Can you work these out from the model? Positions are in its coordinate system, mm. Face numbers are marked on the shaded views. A direction names the side the tool comes from. Round coordinates to 2 decimals unless told otherwise and drop trailing zeros. Order: outer loops, then holes, each group sorted by start corner. A loop starts at its lowest first (then second) coordinate and runs counter-clockwise, first axis right, second up.
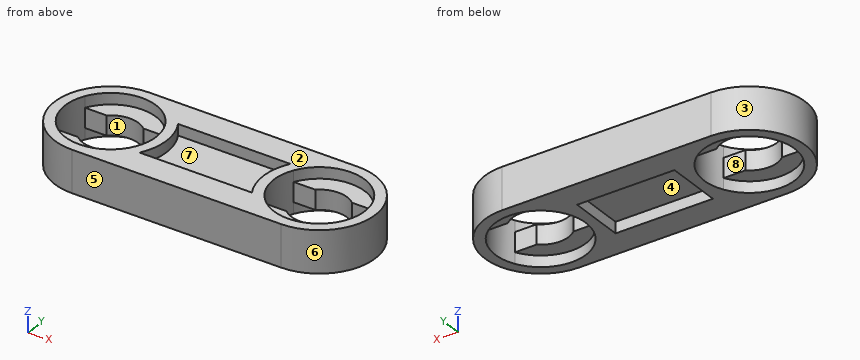
from build123d import *

# Parameters (mm, degrees)
EXTRUDE_1_DEPTH     = 3
CUT_EXTRUDE_1_REACH = 21.647
SKETCH_3_R          = 3.25
CUT_EXTRUDE_2_DEPTH = 0.8
CUT_EXTRUDE_START   = -2.2
SKETCH_3_2_R        = 3.25
CUT_EXTRUDE_3_DEPTH = 0.8
CUT_EXTRUDE_4_DEPTH = 0.8
SKETCH_5_W          = 7
SKETCH_5_H          = 4
CUT_EXTRUDE_5_DEPTH = 0.8


with BuildPart() as part:
    # 草图1 → 凸台-拉伸1 (new body)
    with BuildSketch(Plane.XY):
        with BuildLine():
            Line((0, 4), (15, 4))
            ThreePointArc((15, 4), (19, 0), (15, -4))
            Line((15, -4), (0, -4))
            ThreePointArc((0, -4), (-4, 0), (0, 4))
        make_face()
    extrude(amount=-EXTRUDE_1_DEPTH)

    # 草图2 → 切除-拉伸1 (cut, up to next)
    with BuildSketch(Plane.XY, mode=Mode.PRIVATE) as cut_extrude_1_sk1:
        with BuildLine():
            Line((1.322875656, -1.5), (2.883140649, -1.5))
            ThreePointArc((2.883140649, -1.5), (3.25, 0), (2.883140649, 1.5))
            Line((2.883140649, 1.5), (1.322875656, 1.5))
            ThreePointArc((1.322875656, 1.5), (0, 2), (-1.322875656, 1.5))
            Line((-1.322875656, 1.5), (-2.883140649, 1.5))
            ThreePointArc((-2.883140649, 1.5), (-3.25, 0), (-2.883140649, -1.5))
            Line((-2.883140649, -1.5), (-1.322875656, -1.5))
            ThreePointArc((-1.322875656, -1.5), (0, -2), (1.322875656, -1.5))
        make_face()
    cut_extrude_1_tool1 = extrude(cut_extrude_1_sk1.sketch, amount=-CUT_EXTRUDE_1_REACH, mode=Mode.PRIVATE) & part.part
    cut_extrude_1 = cut_extrude_1_tool1.solids().sort_by_distance((0, 0, 0))[0]
    add(cut_extrude_1, mode=Mode.SUBTRACT)

    # 草图3 → 切除-拉伸2 (cut)
    with BuildSketch(Plane.XY):
        Circle(SKETCH_3_R)
    cut_extrude_2 = extrude(amount=-CUT_EXTRUDE_2_DEPTH, mode=Mode.SUBTRACT)

    # 草图3<2> → 切除-拉伸3 (cut)
    with BuildSketch(Plane.XY.offset(CUT_EXTRUDE_START)):
        Circle(SKETCH_3_2_R)
    cut_extrude_3 = extrude(amount=-CUT_EXTRUDE_3_DEPTH, mode=Mode.SUBTRACT)

    # 镜向1: 切除-拉伸1, 切除-拉伸2, 切除-拉伸3 across plane
    add(cut_extrude_1.mirror(Plane(origin=(7.5, 0, 0), x_dir=(0, 0, 1), z_dir=(1, 0, 0))), mode=Mode.SUBTRACT)
    add(cut_extrude_2.mirror(Plane(origin=(7.5, 0, 0), x_dir=(0, 0, 1), z_dir=(1, 0, 0))), mode=Mode.SUBTRACT)
    add(cut_extrude_3.mirror(Plane(origin=(7.5, 0, 0), x_dir=(0, 0, 1), z_dir=(1, 0, 0))), mode=Mode.SUBTRACT)

    # 草图4 → 切除-拉伸4 (cut)
    with BuildSketch(Plane.XY):
        with BuildLine():
            Line((3.464101615, 2), (11.535898385, 2))
            ThreePointArc((11.535898385, 2), (11, 0), (11.535898385, -2))
            Line((11.535898385, -2), (3.464101615, -2))
            ThreePointArc((3.464101615, -2), (4, 0), (3.464101615, 2))
        make_face()
    extrude(amount=-CUT_EXTRUDE_4_DEPTH, mode=Mode.SUBTRACT)

    # 草图5 → 切除-拉伸5 (cut)
    with BuildSketch(Plane(origin=(0, 0, -3), x_dir=(-1, 0, 0), z_dir=(0, 0, -1))):
        with Locations((-7.5, 0)):
            Rectangle(SKETCH_5_W, SKETCH_5_H)
    extrude(amount=-CUT_EXTRUDE_5_DEPTH, mode=Mode.SUBTRACT)


solid = part.part
(1) If we mould it in two halves opening along Y, with no side actions, what happens to the marked faces 1, 2 and 3? For each: pulls with the +Y half, pulls with the -Y half, needs draft (parallel to the pull), parting line crosses it, or undercut.
(2) I want a section at C-C, the plane x = -0.5. List the corners of the cut face in (y, z) for me.
(3) Please list where these lines run through material, in increasing order: probe 1 along X at (y, z) = (-2.25, -2.4); probe 2 along Y at (x, z) = (6.75, -2.3); probe 3 along X at (y, z) = (0.5, -1.3).
(4) On a 3-axis mill with a long thin cutter (end or side, diameter ignored), from which of +Z, -Z, +X, -X, +Y, -Y can I reach the whole of each face in a straight line? I mean the marked faces 4, 5, 6, 7 and 8. Say none if no direction works.
(5) I want a section at D-D, the plane z = -1.35. List the corners of the cut face in (x, y) for me.
(6) I'm going to push flat-ended pins straight in: pin 1 Ø1.9 at (x, y) = (15.5, -2.5) entering from +Z; pin 2 Ø0.5 at (x, y) = (15.5, 2) entering from -Z; pin 3 Ø0.7 at (x, z) = (-2.5, -1.5) entering from -Y; pin 4 Ø0.5 at (x, y) = (0.5, 2.5) entering from +Z. Where does each tip first touch, or does it pass through?
(7) I want a section at B-B, the plane z = -0.4. List the corners of the cut face in (x, y) for me, plus the area to 3 significant figures.
(8) I want a section at A-A, the plane y = 0. List the corners of the cut face in (x, z) for me, plus the area to 3 significant figures.
Ans:
1. face 1: undercut
1. face 2: needs draft
1. face 3: parting line crosses it
2. outline: (-3.97, -3) - (-3.21, -3) - (-3.21, -2.2) - (-1.94, -2.2) - (-1.94, -0.8) - (-3.21, -0.8) - (-3.21, 0) - (-3.97, 0) - close; (1.94, -2.2) - (3.21, -2.2) - (3.21, -3) - (3.97, -3) - (3.97, 0) - (3.21, 0) - (3.21, -0.8) - (1.94, -0.8) - close
3. probe 1: x = -3.31 to -2.35, 2.35 to 12.65, 17.35 to 18.31
3. probe 2: y = -4 to -2, 2 to 4
3. probe 3: x = -3.97 to -3.21, 3.21 to 11.79, 18.21 to 18.97
4. face 4: -Z
4. face 5: +Z, -Z, +X, -X, -Y
4. face 6: +Z, -Z, +X
4. face 7: +Z
4. face 8: +Z, -Z
5. outline: (0, -4) - (15, -4) arc R4 ccw to (15, 4) - (0, 4) arc R4 ccw to start; hole (-2.88, -1.5) - (-1.32, -1.5) arc R2 ccw to (1.32, -1.5) - (2.88, -1.5) arc R3.25 ccw to (2.88, 1.5) - (1.32, 1.5) arc R2 ccw to (-1.32, 1.5) - (-2.88, 1.5) arc R3.25 ccw to start; hole (12.12, -1.5) - (13.68, -1.5) arc R2 ccw to (16.32, -1.5) - (17.88, -1.5) arc R3.25 ccw to (17.88, 1.5) - (16.32, 1.5) arc R2 ccw to (13.68, 1.5) - (12.12, 1.5) arc R3.25 ccw to start
6. pin 1: stops at z = 0
6. pin 2: stops at z = -2.2
6. pin 3: stops at y = -3.37
6. pin 4: stops at z = -0.8
7. outline: (0, -4) - (15, -4) arc R4 ccw to (15, 4) - (0, 4) arc R4 ccw to start; hole circle Ø6.5 at (0, 0); hole (3.46, -2) - (11.54, -2) arc R4 cw to (11.54, 2) - (3.46, 2) arc R4 cw to start; hole circle Ø6.5 at (15, 0)
7. area: 74.5 mm2
8. outline: (-4, -3) - (-3.25, -3) - (-3.25, 0) - (-4, 0) - close; (3.25, -3) - (4, -3) - (4, -2.2) - (11, -2.2) - (11, -3) - (11.75, -3) - (11.75, 0) - (11, 0) - (11, -0.8) - (4, -0.8) - (4, 0) - (3.25, 0) - close; (18.25, -3) - (19, -3) - (19, 0) - (18.25, 0) - close
8. area: 18.8 mm2
